Part model, mm, in its own coordinate system. Face numbers are marked on the shaded views. A direction names the side the tool comes from. Round coordinates to 2 decimals unless told otherwise and drop trailing zeros. Order: outer loops, then holes, each group sorted by start corner. A loop starts at its lowest first (then second) coordinate and runs counter-clockwise, first axis right, second up. Notation, with made-up numbers: (51.25, 60) - (66.25, 60) arc R27 ccw to (66.25, 98) - close; hole circle Ø1 at (-38, 55). An arc over 180 degrees is marked (long way). Answer as a JSON object with one key per item and string values.
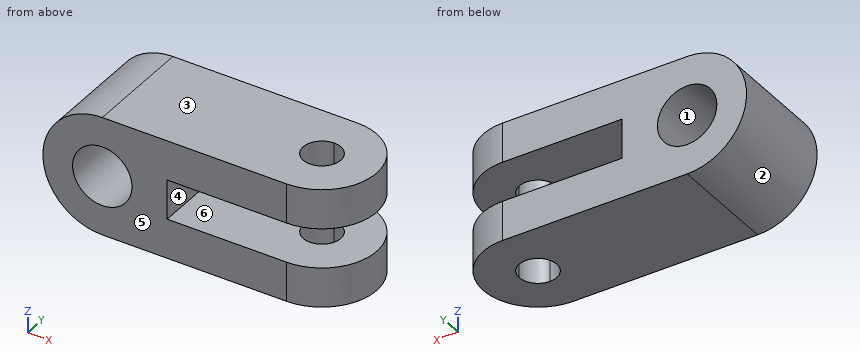
```python
from build123d import *

# Parameters (mm, degrees)
F3_DEPTH = 44.196
F1_W     = 64.77
F1_H     = 14.732
F2_R     = 11.049
F4_DEPTH = 25.4
F2_R_2   = 22.098
F5_DEPTH = 20.32


with BuildPart() as f3:
    # F0 (on Top) → F3 (new body)
    with BuildSketch(Plane.XY):
        with BuildLine():
            Line((32.224336, 20.32), (-36.355664, 20.32))
            Line((-36.355664, 20.32), (-36.355664, -20.32))
            Line((-36.355664, -20.32), (32.224336, -20.32))
            Line((32.224336, -20.32), (32.224336, -6.985))
            ThreePointArc((32.224336, -6.985), (25.239336, 0), (32.224336, 6.985))
            Line((32.224336, 6.985), (32.224336, 20.32))
        make_face()
        with BuildLine():
            ThreePointArc((32.224336, -20.32), (52.544336, 0), (32.224336, 20.32))
            Line((32.224336, 20.32), (32.224336, 6.985))
            ThreePointArc((32.224336, 6.985), (37.163477, 4.939141), (39.209336, 0))
            ThreePointArc((39.209336, 0), (37.163477, -4.939141), (32.224336, -6.985))
            Line((32.224336, -6.985), (32.224336, -20.32))
        make_face()
    extrude(amount=F3_DEPTH)

    # F1 (on Front) + F2 (on Front) → F4 (cut, symmetric)
    with BuildSketch(Plane.XZ):
        with Locations((20.159336, 22.098)):
            Rectangle(F1_W, F1_H)
    with BuildSketch(Plane.XZ):
        with Locations((-36.355664, 22.098)):
            Circle(F2_R)
    extrude(amount=F4_DEPTH, both=True, mode=Mode.SUBTRACT)

    # F2 (on Front) → F5 (join, symmetric)
    with BuildSketch(Plane.XZ):
        with Locations((-36.355664, 22.098)):
            Circle(F2_R_2)
        with Locations((-36.355664, 22.098)):
            Circle(F2_R, mode=Mode.SUBTRACT)
    extrude(amount=F5_DEPTH, both=True)


solid = f3.part
```
Item 1: Cut at C-C (z = 13). Write the cut outline in (x, y) (3 decimals), plus the area to 3 significant figures.
Taken from the geometry:
{"outline": "(-56.494, -20.32) - (-42.625, -20.32) - (-42.625, 20.32) - (-56.494, 20.32) - close; (-30.086, -20.32) - (32.224, -20.32) arc R20.32 ccw to (32.224, 20.32) - (-30.086, 20.32) - close; hole circle Ø13.97 at (32.224, 0)", "area": "3,590 mm2"}
Item 2: Cut at D-D (y = -9.5). Write the cut outline in (x, z), plus the area to 3 significant figures.
Taken from the geometry:
{"outline": "(-36.36, 0) - (50.19, 0) - (50.19, 14.73) - (-12.23, 14.73) - (-12.23, 29.46) - (50.19, 29.46) - (50.19, 44.2) - (-36.36, 44.2) arc R22.1 ccw to start; hole circle Ø22.1 at (-36.36, 22.1)", "area": "3,290 mm2"}
Item 3: Cut at B-B (y = 4). Write the cut outline in (x, z), plus the area to 3 significant figures.
Taken from the geometry:
{"outline": "(-36.36, 0) - (26.5, 0) - (26.5, 14.73) - (-12.23, 14.73) - (-12.23, 29.46) - (26.5, 29.46) - (26.5, 44.2) - (-36.36, 44.2) arc R22.1 ccw to start; (37.95, 0) - (52.15, 0) - (52.15, 14.73) - (37.95, 14.73) - close; (37.95, 29.46) - (52.15, 29.46) - (52.15, 44.2) - (37.95, 44.2) - close; hole circle Ø22.1 at (-36.36, 22.1)", "area": "3,010 mm2"}
Item 4: Cut at A-A (x = 10). Write the cut outline in (y, z).
Taken from the geometry:
{"outline": "(-20.32, 0) - (20.32, 0) - (20.32, 14.73) - (-20.32, 14.73) - close; (-20.32, 29.46) - (20.32, 29.46) - (20.32, 44.2) - (-20.32, 44.2) - close"}
Item 5: Two-plate mould, pull along X, no slides. Class the marked faces 1, 2, 3 and 4: pulls with the +X half, pulls with the -X half, needs draft (parallel to the pull), parting line crosses it, or undercut.
Taken from the geometry:
{"face 1": "undercut", "face 2": "pulls with the -X half", "face 3": "needs draft", "face 4": "pulls with the +X half"}
Item 6: Drop flat-ended pins along their axis: P1, Ø7.5, axis at y = 0, z = 19, coming from the +X side; P2, Ø8, axis at y = 6.5, z = 39, coming from the +X side; P3, Ø5, axis at y = 12, z = 9.5, coming from the -X side; P4, Ø3, axis at x = -33, y = -0.5, coming from the -Z side. Give the stop position or say it passes through.
Taken from the geometry:
{"P1": "x = -12.23", "P2": "x = 52.39", "P3": "x = -56.01", "P4": "z = 0"}
Item 7: Tool access for the marked faces 5 and 6: list every direction of +Z, -Z, +X, -X, +Y, -Y with a clear straight run to the whole face (end or side of a thin tool).
Taken from the geometry:
{"face 5": "+Z, -Z, +X, -X, -Y", "face 6": "+X, +Y, -Y"}
Item 8: Probe L1, parallel to Z at x = -1.5, y = -18; L2, parallel to X at y = 11, z = 22.5; L3, parallel to Y at x = 31, z = 37. List the from-to ranges inside material, lowest first. Write a range as from..to.
Taken from the geometry:
{"L1": "0..14.73, 29.46..44.2", "L2": "-58.45..-47.4, -25.31..-12.23", "L3": "-20.32..-6.88, 6.88..20.32"}
